Source: CAD feature listing. Evaluate the final solid. Frame: model axes, mm. A direction names the side the tool comes from. Give positions to 0.01 mm unless a question says otherwise; leave off trailing zeros. Write each loop counter-clockwise with the first axis right and the second up, starting at its lowest first coordinate (ties: lowest second). Pieces come first, ordered by that corner, then holes. Notation, with made-up numbers: M 72.5,76.25 L 95.5,76.25 A35 cw 95.5,111.25 Z; hole C 52,-34.75 d2. An arc over 180 degrees is marked long. Use CSV: the item, a comma, the result in double quotes. Start each with the question number.
Autodesk Inventor part; units mm, degrees
ref_plane "YZ Plane" through (0, 0, 0) normal (1, 0, 0) x (0, 1, 0)
ref_plane "XZ Plane" through (0, 0, 0) normal (0, 1, 0) x (-1, 0, 0)
ref_plane "XY Plane" through (0, 0, 0) normal (0, 0, 1) x (1, 0, 0)
sketch "Sketch1" plane through (0, 0, 0) normal (0, 0, 1) x (1, 0, 0)
  circle A0 centre (0, 0) radius 3.429
  dimension "head_dia" = 6.858
extrude "Extrusion1" add sketch "Sketch1" against normal blind 4.1656
sketch "Sketch2" plane through (0, 0, -4.1656) normal (0, 0, -1) x (-1, 0, 0)
  circle A0 centre (0, 0) radius 2.0828
  dimension "body_dia" = 4.1656
extrude "Extrusion2" add sketch "Sketch2" along normal blind 6.35
sketch "Sketch3" plane through (0, 0, 0) normal (0, 0, 1) x (1, 0, 0)
  line L0 (2.0622, 0) -> (1.0311, -1.7859)
  line L1 (1.0311, -1.7859) -> (-1.0311, -1.7859)
  line L2 (-1.0311, -1.7859) -> (-2.0622, 0)
  line L3 (-2.0622, 0) -> (-1.0311, 1.7859)
  line L4 (-1.0311, 1.7859) -> (1.0311, 1.7859)
  line L5 (1.0311, 1.7859) -> (2.0622, 0)
  point P0 (0, 0)
  point P1 (0, 0)
  dimension "allen" = 3.5719
extrude "Extrusion3" cut sketch "Sketch3" against normal blind 1.9558
properties part number "shcs-8-0250"
1. Section A-A on x = 0. Return loops of the section in (y, z), then the cut area to 3 significant figures.
2. Access query for faces 1 (the flat face through (-0.05, -2.24, -4.166)), 2 (the flat face through (0, 0, -10.516)), 3 (the flat face through (0, 0, -1.956)). Directions: +Z, -Z, +X, -X, +Y, -Y. A direction counts if a zero-diameter tool reaches every point of the face in a straight line with its end or side. Return the directions, or none.
3. Section B-B on z = -8.75. Return loops of the section in (x, y), then the cut area to 3 significant figures.
4. First-contact query: pin 1 (1 mm diameter, centred on x = 0, z = -9, fed in from +Y); pin 2 (1 mm diameter, centred on x = 1, y = 2.5, fed in from -Z); pin 3 (1.1 mm diameter, centred on x = 0.5, y = -0.5, fed in from +Z). Flat tips, straight axial feed; report the tip coordinate or a pass-through.
5. Line query: probe 1 along Z at (x, y) = (3, -1.5); probe 2 along Z at (x, y) = (0.75, -0.5); probe 3 along X at (y, z) = (0.25, -1.5). Output: solid intervals per line, ascending.
6. Section C-C on x = 0.75. Return loops of the section in (y, z).
7. Section D-D on y = -3. Return loops of the section in (x, z), then the cut area to 3 significant figures.
8. Pull-direction query (Y, two-part tool) for faces 4 (the cylindrical face through (-1.987, -0.626, -7.296)), 5 (the flat face through (0, 1.786, -1)), 6 (the flat face through (1.5, -1.5, 0)); classes: released by +Y, released by -Y, zero draft, split by the parting line, or undercut.
Resolved:
1,outline,"M -3.43,-4.17 L -2.08,-4.17 L -2.08,-10.52 L 2.08,-10.52 L 2.08,-4.17 L 3.43,-4.17 L 3.43,0 L 1.79,0 L 1.79,-1.96 L -1.79,-1.96 L -1.79,0 L -3.43,0 Z"
1,area,"48.0 mm2"
2,face 1,"-Z"
2,face 2,"-Z, +X, -X, +Y, -Y"
2,face 3,"+Z"
3,outline,"C 0,0 d4.17"
3,area,"13.6 mm2"
4,pin 1,"stops at y = 2.08"
4,pin 2,"stops at z = -4.17"
4,pin 3,"stops at z = -1.96"
5,probe 1,"z = -4.17 to 0"
5,probe 2,"z = -10.52 to -1.96"
5,probe 3,"x = -3.42 to -1.92, 1.92 to 3.42"
6,outline,"M -3.35,-4.17 L -1.94,-4.17 L -1.94,-10.52 L 1.94,-10.52 L 1.94,-4.17 L 3.35,-4.17 L 3.35,0 L 1.79,0 L 1.79,-1.96 L -1.79,-1.96 L -1.79,0 L -3.35,0 Z"
7,outline,"M -1.66,-4.17 L 1.66,-4.17 L 1.66,0 L -1.66,0 Z"
7,area,"13.8 mm2"
8,face 4,"split by the parting line"
8,face 5,"undercut"
8,face 6,"zero draft"
